```python
from build123d import *

# Parameters (mm, degrees)
BASE_FLANGE1_DEPTH          = 110
F_3_0MM_PRESS_DOWEL_HOLE1_D = 3


# Sheet-metal steps are written as plain solids
with BuildPart() as part:
    # Sketch1 → Base-Flange1 (new body)
    with BuildSketch(Plane(origin=(0, 0, 0), x_dir=(1, 0, 0), z_dir=(0, 1, 0))):
        with BuildLine():
            Line((0, 0), (-2.270295707, 109.460685851))
            ThreePointArc((-2.270295707, 109.460685851), (-2.412240672, 109.880329075), (-2.769212645, 110.142664393))
            Line((-2.769212645, 110.142664393), (-16.479732829, 114.813260902))
            Line((-16.479732829, 114.813260902), (-15.996041521, 116.233135093))
            Line((-15.996041521, 116.233135093), (-2.285521337, 111.562538584))
            ThreePointArc((-2.285521337, 111.562538584), (-1.201617569, 110.765987985), (-0.770618236, 109.491790273))
            Line((-0.770618236, 109.491790273), (1.49967747, 0.031104422))
            Line((1.49967747, 0.031104422), (0, 0))
        make_face()
    extrude(amount=BASE_FLANGE1_DEPTH)

    # Ø3.0mm Press Dowel Hole1 (through all)
    with Locations(Plane(origin=(33.81524251, 0, -99.264529514), x_dir=(-0.9465827940969574, 0, -0.32246087192029516), z_dir=(0.32246087192029516, 0, -0.9465827940969574))):
        with Locations((47.622215766, 10), (47.622215766, 100)):
            Hole(F_3_0MM_PRESS_DOWEL_HOLE1_D / 2)


solid = part.part
```
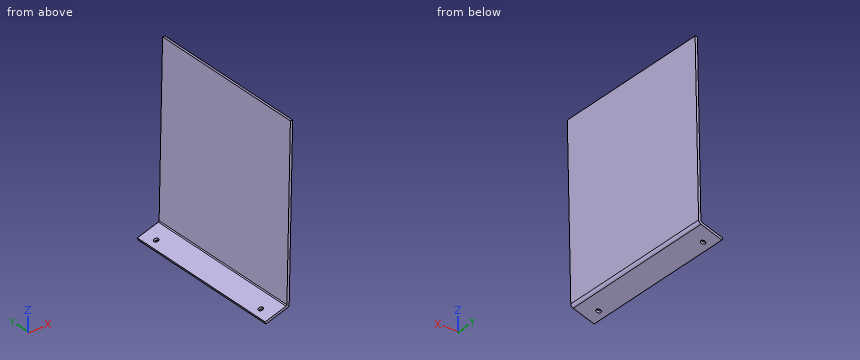
For this review, take the finished solid that the model builds, in its own axes (mm). Round coordinates to 2 decimals unless told otherwise and drop trailing zeros. Write each loop counter-clockwise with the first axis right and the second up, starting at its lowest first coordinate (ties: lowest second). Pieces come first, ordered by that corner, then holes. Notation, with made-up numbers: (80.5, 62.5) - (123.5, 62.5) arc R29 cw to (123.5, 88.5) - close; hole circle Ø1 at (-8, 29). An arc over 180 degrees is marked (long way). Write each question's results on one line, items separated by ' | '.
Item 1: Take a section at B-B on z = -24. State the section outline as (x, y) points, then the cut area to 3 significant figures.
Calculated:
outline: (-0.5, 0) - (1, 0) - (1, 110) - (-0.5, 110) - close | area: 165 mm^2
Item 2: For pin 1 (12 mm diameter, centred on y = 12, z = -90.5, fed in from +X); pin 2 (5 mm diameter, centred on y = 42.5, z = -29.5, fed in from -X); pin 3 (4 mm diameter, centred on y = 61.5, z = -41.5, fed in from +X), all flat-tipped, find the tip position at first contact; note any pin that passes through.
Calculated:
pin 1: stops at x = -0.25 | pin 2: stops at x = -0.66 | pin 3: stops at x = 0.68
Item 3: Take a section at C-C on x = -6.75. State the section outline as (y, z) points, then the cut area to 3 significant figures.
Calculated:
outline: (0, -113.08) - (110, -113.08) - (110, -111.5) - (0, -111.5) - close | area: 174 mm^2
Item 4: To check wall thickness, follow line 1 along X through (y, z) = (64, -57); line 2 along X through (y, z) = (86, -101); line 3 along Z through (x, y) = (-8.25, 9). State the ranges of each line that lie inside material, in increasing order. Write a range as from..to.
Calculated:
line 1: x = -1.18..0.32 | line 2: x = -2.09..-0.59 | line 3: z = -113.59..-112.01
Item 5: Take a section at A-A on y = 63.5. State the section outline as (x, z) points.
Calculated:
outline: (-16.48, -114.81) - (-16, -116.23) - (-2.29, -111.56) arc R2.24 ccw to (-0.77, -109.49) - (1.5, -0.03) - (0, 0) - (-2.27, -109.46) arc R0.74 cw to (-2.77, -110.14) - close
